Check sheet for the modelled part. Datum: model origin and axes. Units: mm. Face numbers are marked on the shaded views. A direction names the side the tool comes from. Give positions to 0.01 mm unless a question says otherwise; leave off trailing zeros. Write each loop counter-clockwise with the first axis right and the second up, starting at its lowest first coordinate (ties: lowest second). Pieces come first, ordered by that corner, then holes. Notation, with made-up numbers: M 26,14 L 72,14 A23 cw 72,24 Z; hole C -9.75,-27.75 d4. An arc over 180 degrees is marked long. Use CSV: the item, a comma, the result in double quotes. Start each with the question number.
1. Scan lines: line 1 (Y direction, x = -63, z = 50); line 2 (X direction, y = 11, z = 68); line 3 (Z direction, x = -12, y = 15). Record each from-to range of solid material in increasing order.
2. Cross-section at D-D, the plane y = 33. Enter the section's corners in (x, z).
3. Access from +Z, -Z, +X, -X, +Y, -Y to the whole of each face (thin tool, end or side, straight path). Record for the marked faces 4, 5, 6, 7 and 8.
4. Cross-section at C-C, the plane z = 74. Enter the section's corners in (x, y), and give its area (3 significant figures).
5. Mould release check, pull along X, two halves, no side actions. Record for the marked faces 1, 2 and 3: +X half, -X half, draft (parallel to the pull), parting line (faces both ways), or undercut.
6. Cross-section at A-A, the plane y = 15. Enter the section's corners in (x, z), and give its area (3 significant figures).
7. Depth check by flat-ended pin: P1, Ø5, axis at x = -9, z = 40, coming from the -Y side; P2, Ø12, axis at x = -17, y = -9, coming from the +Z side; P3, Ø1.5, axis at x = -18.5, z = 35, coming from the +Y side; P4, Ø12, axis at x = -34.5, y = -11.5, coming from the +Z side. Enter the tip coordinate at first touch or a pass-through.
8. Cross-section at B-B, the plane x = -10. Enter the section's corners in (y, z).
Solid Edge part; units mm, degrees
sketch "Sketch1" plane through (0, 0, 0) normal (1, 0, 0) x (0, 1, 0)
  line L0 (45, 0) -> (45, 50)
  line L1 (-45, 0) -> (45, 0)
  line L2 (-45, 24) -> (-45, 0)
  line L3 (-15, 24) -> (-45, 24)
  line L4 (-15, 50) -> (-15, 24)
  arc A0 (-15, 50) -> (45, 50) centre (15, 50) cw
extrude "ProtrusiónExtruida_1" add sketch "Sketch1" against normal blind 70
sketch "Sketch2" plane through (-35, -15, 37) normal (0, -1, 0) x (1, 0, 0)
  line L0 (-19, -13) -> (-19, 43)
  line L1 (-19, 43) -> (19, 43)
  line L2 (19, 43) -> (19, -13)
  line L3 (19, -13) -> (-19, -13)
extrude "VaciadoExtruido_1" cut sketch "Sketch2" against normal blind 60
hole "Agujero_1" at (0, 15, 50) direction (-1, 0, 0) diameter 28 end through all
sketch "Sketch3" plane through (-35, 0, 24) normal (0, 0, 1) x (0, 1, 0)
  line L0 (-45, 21) -> (-27, 21)
  line L1 (-27, 21) -> (-27, -21)
  line L2 (-27, -21) -> (-45, -21)
  line L3 (-45, -21) -> (-45, 21)
extrude "VaciadoExtruido_2" cut sketch "Sketch3" against normal blind 24
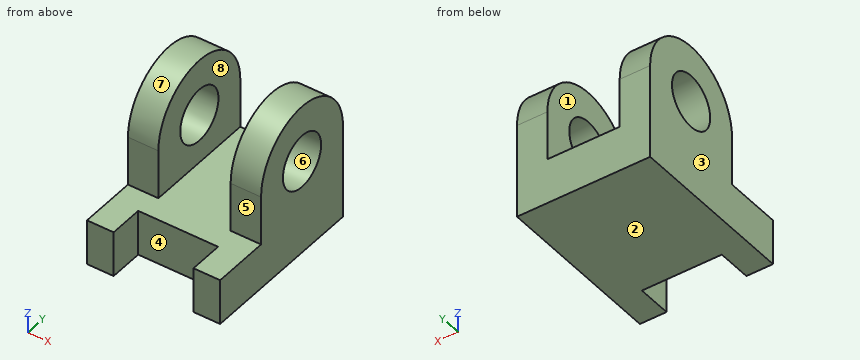
Worked answers:
1,line 1,"y = -15 to 1, 29 to 45"
1,line 2,"x = -70 to -54, -16 to 0"
1,line 3,"z = 0 to 36, 64 to 80"
2,outline,"M -70,0 L 0,0 L 0,74 L -16,74 L -16,24 L -54,24 L -54,74 L -70,74 Z"
3,face 4,"+Z, -Z, -Y"
3,face 5,"+Z, +X, -X, -Y"
3,face 6,"+X, -X"
3,face 7,"+Z, +X, -X"
3,face 8,"+Z, +Y, -Y"
4,outline,"M -70,-3 L -54,-3 L -54,33 L -70,33 Z; M -16,-3 L 0,-3 L 0,33 L -16,33 Z"
4,area,"1,150 mm^2"
5,face 1,"undercut"
5,face 2,"draft"
5,face 3,"-X half"
6,outline,"M -70,0 L 0,0 L 0,36 L -16,36 L -16,24 L -54,24 L -54,36 L -70,36 Z; M -70,64 L -54,64 L -54,80 L -70,80 Z; M -16,64 L 0,64 L 0,80 L -16,80 Z"
6,area,"2,580 mm^2"
7,P1,"stops at y = -15"
7,P2,"stops at z = 73.94"
7,P3,"passes through"
7,P4,"stops at z = 24"
8,outline,"M -45,0 L 45,0 L 45,50 A30 ccw -15,50 L -15,24 L -45,24 Z; hole C 15,50 d28"
